from build123d import *

# Parameters (mm, degrees)
F1_DEPTH = 762
F2_W     = 685.8
F2_H     = 88.9
F2_W_2   = 609.6
F2_H_2   = 101.6
F3_DEPTH = 457.201
F4_W     = 143.9333333333
F4_H     = 304.8
F5_DEPTH = 508


with BuildPart() as f1:
    # F0 (on Right) → F1 (new body)
    with BuildSketch(Plane.YZ):
        with BuildLine():
            ThreePointArc((88.9, 812.8), (26.0382071525, 786.7617928475), (0, 723.9))
            Line((0, 723.9), (457.2, 723.9))
            ThreePointArc((457.2, 723.9), (431.1617928475, 786.7617928475), (368.3, 812.8))
            Line((368.3, 812.8), (88.9, 812.8))
        make_face()
        Polygon((0, 723.9), (0, 0), (63.5, 0), (63.5, 101.6), (393.7, 101.6), (393.7, 0), (457.2, 0), (457.2, 723.9), align=None)
    extrude(amount=F1_DEPTH)

    # F2 (on face) → F3 (cut, through all)
    with BuildSketch(Plane.XZ):
        with Locations((381, 768.35)):
            Rectangle(F2_W, F2_H)
        with Locations((381, 50.8)):
            Rectangle(F2_W_2, F2_H_2)
    extrude(amount=-F3_DEPTH, mode=Mode.SUBTRACT)

    # F4 (on face) → F5 (cut)
    with BuildSketch(Plane.XY.offset(723.9)):
        with Locations((186.2666666667, 228.6)):
            Rectangle(F4_W, F4_H)
        with Locations((381, 228.6)):
            Rectangle(F4_W, F4_H)
        with Locations((575.7333333333, 228.6)):
            Rectangle(F4_W, F4_H)
    extrude(amount=-F5_DEPTH, mode=Mode.SUBTRACT)


solid = f1.part
Here's how the part is built. I have some questions about the finished solid (model axes, mm). A direction names the side the tool comes from. Give positions to 0.01 mm unless a question says otherwise; leave off trailing zeros. Order: outer loops, then holes, each group sorted by start corner. A loop starts at its lowest first (then second) coordinate and runs counter-clockwise, first axis right, second up. Notation, with made-up numbers: (82, 57.25) -> (122, 57.25) arc R30 ccw to (122, 92.25) -> close; hole circle Ø3 at (31, 7.5). An arc over 180 degrees is marked (long way). One line per item, written item: value. Start each with the question number.
1. Will these pins go through, and if not, where does the flat tip stop? pin 1 Ø1 at (x, y) = (361, 120.5) entering from -Z; pin 2 Ø4 at (x, y) = (97.5, 264) entering from +Z.
2. For faces 3 (the face through (723, 393.7, 52)), 4 (the face through (723, 31, 0)), 5 (the face through (38.1, 225, 768)), 6 (the face through (114.3, 226, 473)), 7 (the face through (76.2, 31, 50)), which set-ups out of +Z, -Z, +X, -X, +Y, -Y let a thin tool reach every point of the face, with its end or its side?
3. Imagine slicing it at A-A, the plane z = 387. List the corners of the cut face in (x, y) for me.
4. Imagine slicing it at C-C, the plane y = 177.5. List the corners of the cut face in (x, z) for me, plus the area to 3 significant figures.
5. I need wall thicknesses on probe 1 along X at (y, z) = (100, 358); probe 2 along Y at (x, z) = (426.5, 565.5); probe 3 along X at (y, z) = (282, 729.5). Which ranges of each line are inside material? Lowest first, please. Write a range as from..to.
6. Imagine slicing it at B-B, the plane z = 67.5. List the corners of the cut face in (x, y) for me, plus the area to 3 significant figures.
7. We'd pull the mould along X, two halves only. Please class faces 1 (the face through (38, 393.7, 52)), 2 (the face through (76.2, 425, 50)): released by +X, released by -X, zero draft, split by the parting line, or undercut.
8. Imagine slicing it at D-D, the plane x = 357.5. List the corners of the cut face in (y, z) for me.
Values follow:
1. pin 1: stops at z = 101.6
1. pin 2: stops at z = 723.9
2. face 3: -Z, +X, -X
2. face 4: -Z, +X, -X, +Y, -Y
2. face 5: +Z, +Y, -Y
2. face 6: +Z
2. face 7: -Z, +Y, -Y
3. outline: (0, 0) -> (762, 0) -> (762, 457.2) -> (0, 457.2) -> close; hole (114.3, 76.2) -> (258.23, 76.2) -> (258.23, 381) -> (114.3, 381) -> close; hole (309.03, 76.2) -> (452.97, 76.2) -> (452.97, 381) -> (309.03, 381) -> close; hole (503.77, 76.2) -> (647.7, 76.2) -> (647.7, 381) -> (503.77, 381) -> close
4. outline: (0, 101.6) -> (762, 101.6) -> (762, 812.8) -> (723.9, 812.8) -> (723.9, 723.9) -> (647.7, 723.9) -> (647.7, 215.9) -> (503.77, 215.9) -> (503.77, 723.9) -> (452.97, 723.9) -> (452.97, 215.9) -> (309.03, 215.9) -> (309.03, 723.9) -> (258.23, 723.9) -> (258.23, 215.9) -> (114.3, 215.9) -> (114.3, 723.9) -> (38.1, 723.9) -> (38.1, 812.8) -> (0, 812.8) -> close
4. area: 262,000 mm2
5. probe 1: x = 0..114.3, 258.23..309.03, 452.97..503.77, 647.7..762
5. probe 2: y = 0..76.2, 381..457.2
5. probe 3: x = 0..38.1, 723.9..762
6. outline: (0, 0) -> (76.2, 0) -> (76.2, 63.5) -> (0, 63.5) -> close; (0, 393.7) -> (76.2, 393.7) -> (76.2, 457.2) -> (0, 457.2) -> close; (685.8, 0) -> (762, 0) -> (762, 63.5) -> (685.8, 63.5) -> close; (685.8, 393.7) -> (762, 393.7) -> (762, 457.2) -> (685.8, 457.2) -> close
6. area: 19,400 mm2
7. face 1: zero draft
7. face 2: undercut
8. outline: (0, 101.6) -> (457.2, 101.6) -> (457.2, 723.9) -> (381, 723.9) -> (381, 215.9) -> (76.2, 215.9) -> (76.2, 723.9) -> (0, 723.9) -> close
